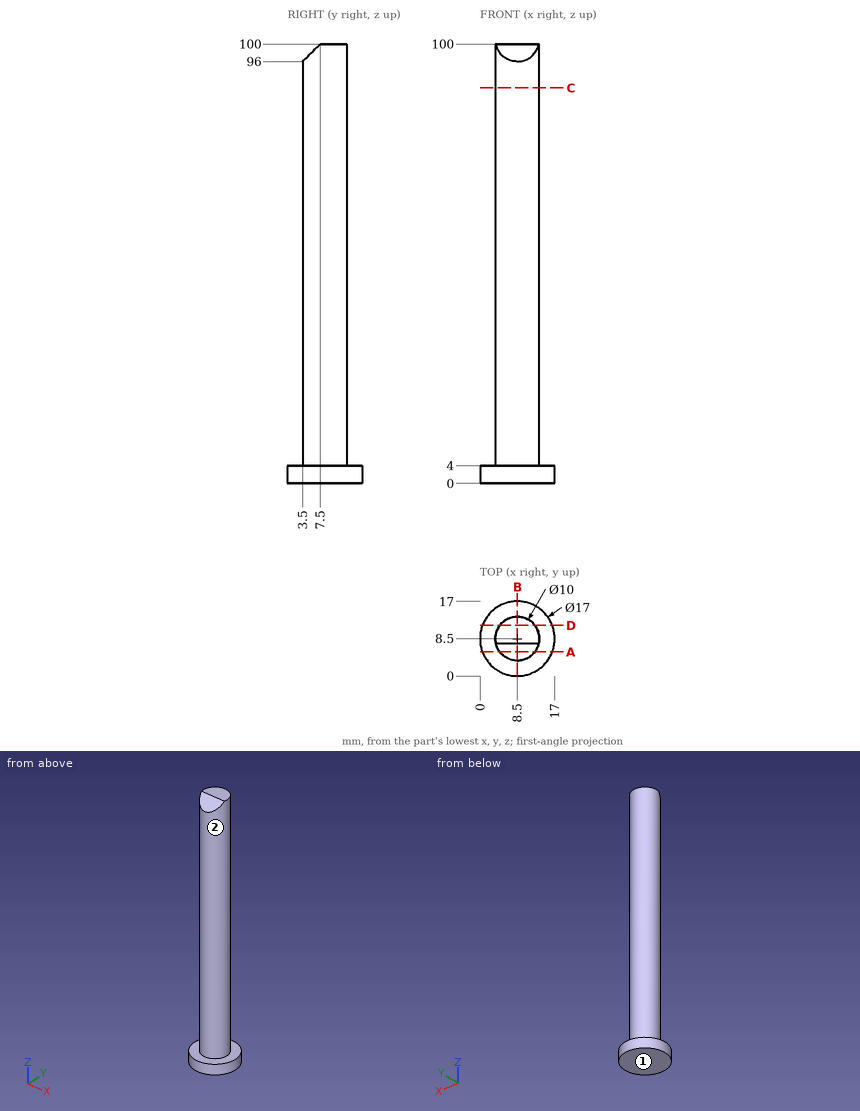
Print and shaded views of the part. All mm, measured from the part's lowest x, y and z. A direction names the side the tool comes from. Coordinates: 2 decimals unless noted, no trailing zeros. Loops run counter-clockwise (first coordinate to the right, second up) from the corner with the lowest first, then second, coordinate; pieces in that order, holes last. Notation, with made-up numbers: M 69.25,42 L 128.25,42 A28 cw 128.25,80 Z; hole C 11,75.5 d8. An arc over 180 degrees is marked long. Use a Markdown table: item, result. Add a question column.
Q1. Cut at C-C (z = 90). Write the cut outline in (x, y), and give its area (3 significant figures).
Q2. Cut at B-B (x = 8.5). Write the cut outline in (y, z).
Q3. Probe L1, parallel to Z at x = 4.75, y = 12.5; L2, parallel to X at y = 4.75, z = 45; L3, parallel to X at y = 5, z = 60.5. List the from-to ranges inside material, lowest first.
Q4. Cut at D-D (y = 11.5). Write the cut outline in (x, z), and give its area (3 significant figures).
Q5. Pin check, flat tips, straight feed: P1, Ø6, axis at x = 5, y = 6.5, coming from the +Z side; P2, Ø5, axis at x = 9, z = 25.5, coming from the +Y side; P3, Ø2, axis at y = 11.5, z = 16.5, coming from the -X side; P4, Ø2, axis at y = 4, z = 19.5, coming from the -X side. Stop position of each tip, or through.
Q6. Cut at A-A (y = 5.5). Write the cut outline in (x, z), and give its area (3 significant figures).
Q7. Which spindle directions (+Z, -Z, +X, -X, +Y, -Y) get a long thin tool onto all of the face, cutting with end or side? Do the marked faces 1 and 2. Say none if no direction does.
Worked out:
| question | item | result |
|---|---|---|
| 1 | outline | C 8.5,8.5 d10 |
| 1 | area | 78.5 mm2 |
| 2 | outline | M 0,0 L 17,0 L 17,4 L 13.5,4 L 13.5,100 L 7.5,100 L 3.5,96 L 3.5,4 L 0,4 Z |
| 3 | L1 | z = 0 to 4 |
| 3 | L2 | x = 5.19 to 11.81 |
| 3 | L3 | x = 4.93 to 12.07 |
| 4 | outline | M 0.55,0 L 16.45,0 L 16.45,4 L 12.5,4 L 12.5,100 L 4.5,100 L 4.5,4 L 0.55,4 Z |
| 4 | area | 832 mm2 |
| 5 | P1 | stops at z = 100 |
| 5 | P2 | stops at y = 13.5 |
| 5 | P3 | stops at x = 3.92 |
| 5 | P4 | stops at x = 4.93 |
| 6 | outline | M 0.55,0 L 16.45,0 L 16.45,4 L 12.5,4 L 12.5,98 L 4.5,98 L 4.5,4 L 0.55,4 Z |
| 6 | area | 816 mm2 |
| 7 | face 1 | -Z, +X, -X, +Y, -Y |
| 7 | face 2 | +Z |
